Read the model definition and answer for the solid it produces. Units are mm, in the model's axes. Face numbers are marked on the shaded views. A direction names the side the tool comes from. Coordinates: 2 decimals unless noted, no trailing zeros. Write each loop counter-clockwise with the first axis right and the second up, starting at its lowest first coordinate (ties: lowest second). Pieces come first, ordered by that corner, then holes. Notation, with made-up numbers: (79.25, 71) - (126.25, 71) arc R25 ccw to (126.25, 84) - close; hole circle Ø10 at (58, -1.5). An arc over 180 degrees is marked (long way). Return JSON: item names as keys, results as strings.
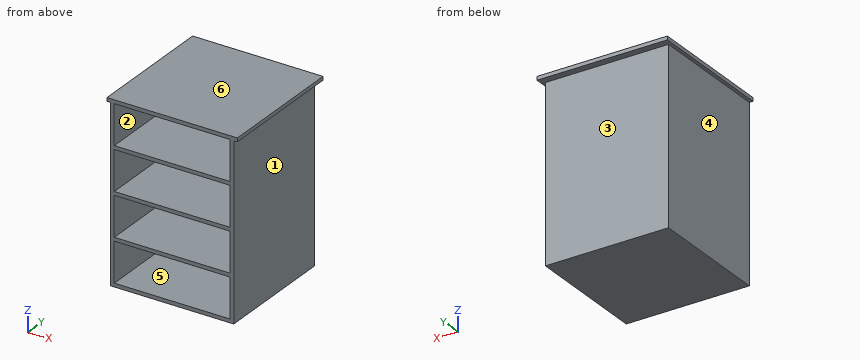
```python
from build123d import *

# Parameters (mm, degrees)
F0_W     = 863.6
F0_H     = 863.6
F1_DEPTH = 1219.2
F2_W     = 863.6
F2_H     = 863.6
F3_DEPTH = 25.4
F4_W     = 812.8
F4_H     = 279.4
F5_DEPTH = 762


with BuildPart() as f1:
    # F0 (on Top) → F1 (new body)
    with BuildSketch(Plane.XY):
        with Locations((435.757004, 431.8)):
            Rectangle(F0_W, F0_H)
    extrude(amount=F1_DEPTH)

    # F2 (on face) → F3 (join)
    with BuildSketch(Plane.XY.offset(1219.2)):
        Polygon((867.557004, 863.6), (867.557004, 0), (892.957004, 0), (892.957004, 914.4), (-21.442996, 914.4), (-21.442996, 0), (3.957004, 0), (3.957004, 863.6), align=None)
        with Locations((435.757004, 431.8)):
            Rectangle(F2_W, F2_H)
    extrude(amount=F3_DEPTH)

    # F4 (on face) → F5 (cut)
    with BuildSketch(Plane.XZ):
        with Locations((435.757004, 1079.5)):
            Rectangle(F4_W, F4_H)
        with Locations((435.757004, 774.7)):
            Rectangle(F4_W, F4_H)
        with Locations((435.757004, 469.9)):
            Rectangle(F4_W, F4_H)
        with Locations((435.757004, 165.1)):
            Rectangle(F4_W, F4_H)
    extrude(amount=-F5_DEPTH, mode=Mode.SUBTRACT)


solid = f1.part
```
(1) Straight lines are drawn through the part: line 1 (Z direction, x = 564.5, y = 53); line 2 (X direction, y = 756, z = 986.5); line 3 (Y direction, x = 73, z = 1008). For each, find the intervals that lie inside material, in ascending order. Write a range as from..to.
Answer:
{"line 1": "0..25.4, 304.8..330.2, 609.6..635, 914.4..939.8, 1219.2..1244.6", "line 2": "3.96..29.36, 842.16..867.56", "line 3": "762..863.6"}
(2) A cutting plane is placed at A-A (y = 383.5). Determine the outline of the cut face in (x, z).
Answer:
{"outline": "(-21.44, 1219.2) - (3.96, 1219.2) - (3.96, 0) - (867.56, 0) - (867.56, 1219.2) - (892.96, 1219.2) - (892.96, 1244.6) - (-21.44, 1244.6) - close; hole (29.36, 25.4) - (842.16, 25.4) - (842.16, 304.8) - (29.36, 304.8) - close; hole (29.36, 330.2) - (842.16, 330.2) - (842.16, 609.6) - (29.36, 609.6) - close; hole (29.36, 635) - (842.16, 635) - (842.16, 914.4) - (29.36, 914.4) - close; hole (29.36, 939.8) - (842.16, 939.8) - (842.16, 1219.2) - (29.36, 1219.2) - close"}
(3) A cutting plane is placed at B-B (x = 713.5). Determine the outline of the cut face in (y, z).
Answer:
{"outline": "(0, 0) - (863.6, 0) - (863.6, 1219.2) - (914.4, 1219.2) - (914.4, 1244.6) - (0, 1244.6) - (0, 1219.2) - (762, 1219.2) - (762, 939.8) - (0, 939.8) - (0, 914.4) - (762, 914.4) - (762, 635) - (0, 635) - (0, 609.6) - (762, 609.6) - (762, 330.2) - (0, 330.2) - (0, 304.8) - (762, 304.8) - (762, 25.4) - (0, 25.4) - close"}
(4) Flat-ended cylindrical pins translate along their axes: P1, Ø4, axis at x = 364, z = 995, coming from the +Y side; P2, Ø1.5, axis at y = 257.5, z = 258.5, coming from the -X side; P3, Ø2, axis at x = 398.5, z = 1100, coming from the -Y side. Find the tip coordinate at first contact, or state that the pin passes through.
Answer:
{"P1": "y = 863.6", "P2": "x = 3.96", "P3": "y = 762"}
(5) Which of the six approach directions +Z, -Z, +X, -X, +Y, -Y give full straight-line access (tool end or side, diameter ignored) to the marked faces 5 and 6?
Answer:
{"face 5": "-Y", "face 6": "+Z, +X, -X, +Y, -Y"}
(6) A cutting plane is placed at C-C (z = 822). Determine the outline of the cut face in (x, y).
Answer:
{"outline": "(3.96, 0) - (29.36, 0) - (29.36, 762) - (842.16, 762) - (842.16, 0) - (867.56, 0) - (867.56, 863.6) - (3.96, 863.6) - close"}
(7) Determine the mould class of the marked faces 1, 2, 3 and 4 for opening direction X: +X half, -X half, draft (parallel to the pull), parting line (faces both ways), or undercut.
Answer:
{"face 1": "+X half", "face 2": "undercut", "face 3": "draft", "face 4": "-X half"}
